from build123d import *

# Parameters (mm, degrees)
F0_W      = 88.9
F0_H      = 88.9
F1_DEPTH  = 914.4
F2_W      = 88.9
F2_H      = 38.1
F3_DEPTH  = 1803.4
F4_W      = 88.9
F4_H      = 88.9
F5_DEPTH  = 914.4
F6_W      = 38.1
F6_H      = 88.9
F7_DEPTH  = 1295.4
F8_W      = 88.9
F8_H      = 88.9
F9_DEPTH  = 914.4
F10_W     = 38.1
F10_H     = 88.9
F11_DEPTH = 1295.4
F12_W     = 88.9
F12_H     = 88.9
F13_DEPTH = 914.4
F14_W     = 88.9
F14_H     = 38.1
F15_DEPTH = 1803.4
F16_W     = 1879.6
F16_H     = 1371.6
F17_DEPTH = 12.7
F18_W     = 1955.8
F18_H     = 1447.8
F18_W_2   = 1879.6
F18_H_2   = 1371.6
F19_DEPTH = 88.9


with BuildPart() as f1:
    # F0 (on Front) → F1 (new body)
    with BuildSketch(Plane.XZ):
        Rectangle(F0_W, F0_H)
    extrude(amount=F1_DEPTH)

    # F2 (on face) → F3 (join)
    with BuildSketch(Plane.YZ.offset(44.45)):
        with Locations((-44.45, -25.4)):
            Rectangle(F2_W, F2_H)
    extrude(amount=F3_DEPTH)

    # F4 (on Front) → F5 (join)
    with BuildSketch(Plane.XZ):
        with Locations((1892.3, 0)):
            Rectangle(F4_W, F4_H)
    extrude(amount=F5_DEPTH)

    # F6 (on face) → F7 (join)
    with BuildSketch(Plane(origin=(0, 0, -44.45), x_dir=(1, 0, 0), z_dir=(0, 0, -1))):
        with Locations((1866.9, 44.45)):
            Rectangle(F6_W, F6_H)
    extrude(amount=F7_DEPTH)

    # F8 (on Front) → F9 (join)
    with BuildSketch(Plane.XZ):
        with Locations((1892.3, -1384.3)):
            Rectangle(F8_W, F8_H)
    extrude(amount=F9_DEPTH)

    # F10 (on face) → F11 (join)
    with BuildSketch(Plane(origin=(0, 0, -44.45), x_dir=(1, 0, 0), z_dir=(0, 0, -1))):
        with Locations((25.4, 44.45)):
            Rectangle(F10_W, F10_H)
    extrude(amount=F11_DEPTH)

    # F12 (on Front) → F13 (join)
    with BuildSketch(Plane.XZ):
        with Locations((0, -1384.3)):
            Rectangle(F12_W, F12_H)
    extrude(amount=F13_DEPTH)

    # F14 (on face) → F15 (join)
    with BuildSketch(Plane.YZ.offset(44.45)):
        with Locations((-44.45, -1358.9)):
            Rectangle(F14_W, F14_H)
    extrude(amount=F15_DEPTH)

    # F16 (on Front) → F17 (join)
    with BuildSketch(Plane.XZ):
        with Locations((946.15, -692.15)):
            Rectangle(F16_W, F16_H)
    extrude(amount=-F17_DEPTH)

    # F18 (on Front) → F19 (join)
    with BuildSketch(Plane.XZ):
        with Locations((946.15, -692.15)):
            Rectangle(F18_W, F18_H)
        with Locations((946.15, -692.15)):
            Rectangle(F18_W_2, F18_H_2, mode=Mode.SUBTRACT)
    extrude(amount=-F19_DEPTH)


solid = f1.part
For this review, take the finished solid that the model builds, in its own axes (mm). A direction names the side the tool comes from. Round coordinates to 2 decimals unless told otherwise and drop trailing zeros. Loops run counter-clockwise (first coordinate to the right, second up) from the corner with the lowest first, then second, coordinate; pieces in that order, holes last. Notation, with made-up numbers: (27, 22.5) - (84, 22.5) arc R19 ccw to (84, 56.5) - close; hole circle Ø2 at (19, -7.75). An arc over 180 degrees is marked (long way). One line per item, written item: value. Start each with the question number.
Item 1: For faces 1 (the flat face through (934, -45, -1339.85)), 2 (the flat face through (1885.95, 50, -702)), 3 (the flat face through (1892, -914.4, -1384)), list the 3-axis set-ups (+Z, -Z, +X, -X, +Y, -Y) from which the entire face can be reached by the end or side of a thin tool; tool diameter is ignored.
Item 2: Take a section at C-C (z = -654.5). Give the boundary of the cut face in (x, y).
Item 3: Take a section at A-A (x = 1236.5). Give the boundary of the cut face in (y, z).
Item 4: The part is to be moulded in two halves that separate along Z. For faces 4 (the flat face through (934, -45, -1377.95)), 5 (the flat face through (1885.95, -45, -701)), 6 (the flat face through (-1, -914.4, -1384)), say which applies: +Z half, -Z half, draft (parallel to the pull), parting line (faces both ways), or undercut.
Item 5: For L1, parallel to Z at x = 619.5, y = -64.5; L2, parallel to Z at x = 1228.5, y = 42; L3, parallel to X at y = -632.5, z = -1346, list the stretches that pass through material, from the lowest coordinate up.
Item 6: Clearance check with flat-ended pins moving along their axes: pin 1 Ø8 at (x, z) = (368.5, -889) entering from +Y; pin 2 Ø5 at (x, z) = (1266.5, -884) entering from -Y. State where each tip first meets the part, or that it passes through.
Item 7: Take a section at B-B (y = -777). Give the boundary of the cut face in (x, z), plus the area to 3 significant figures.
Answer below:
1. face 1: -Y
1. face 2: +Y
1. face 3: +Z, -Z, +X, -X, -Y
2. outline: (-31.75, 0) - (6.35, 0) - (6.35, -88.9) - (44.45, -88.9) - (44.45, 0) - (1847.85, 0) - (1847.85, -88.9) - (1885.95, -88.9) - (1885.95, 0) - (1924.05, 0) - (1924.05, 88.9) - (1885.95, 88.9) - (1885.95, 12.7) - (6.35, 12.7) - (6.35, 88.9) - (-31.75, 88.9) - close
3. outline: (-88.9, -1377.95) - (0, -1377.95) - (0, -1416.05) - (88.9, -1416.05) - (88.9, -1377.95) - (12.7, -1377.95) - (12.7, -6.35) - (88.9, -6.35) - (88.9, 31.75) - (0, 31.75) - (0, -6.35) - (-88.9, -6.35) - (-88.9, -44.45) - (0, -44.45) - (0, -1339.85) - (-88.9, -1339.85) - close
4. face 4: -Z half
4. face 5: undercut
4. face 6: draft
5. L1: z = -1377.95 to -1339.85, -44.45 to -6.35
5. L2: z = -1416.05 to -1377.95, -6.35 to 31.75
5. L3: x = -44.45 to 44.45, 1847.85 to 1936.75
6. pin 1: stops at y = 12.7
6. pin 2: stops at y = 0
7. outline: (-44.45, -1428.75) - (44.45, -1428.75) - (44.45, -1339.85) - (-44.45, -1339.85) - close; (-44.45, -44.45) - (44.45, -44.45) - (44.45, 44.45) - (-44.45, 44.45) - close; (1847.85, -1428.75) - (1936.75, -1428.75) - (1936.75, -1339.85) - (1847.85, -1339.85) - close; (1847.85, -44.45) - (1936.75, -44.45) - (1936.75, 44.45) - (1847.85, 44.45) - close
7. area: 31,600 mm2
